Could you check a few things on this drawing? It's one solid part, dimensions in mm from its lowest x, y, z. A direction names the side the tool comes from. Coordinates: 2 decimals unless noted, no trailing zeros. Loops run counter-clockwise (first coordinate to the right, second up) from the corner with the lowest first, then second, coordinate; pieces in that order, holes last. Notation, with made-up numbers: M -38.75,-29 L -26.75,-29 A16 ccw -26.75,-8 Z; hole C -2.75,-16 d11. An arc over 180 degrees is marked long. Use one line per item in the form item = value. Start each with the question number.
(1) Imagine slicing it at A-A, the plane z = 10. Please give me the cut outline in (x, y), and give its area (3 significant figures).
(2) Please list where these lines run through material, in increasing order: L1, parallel to Y at x = 7.07, z = 31.5; L2, parallel to Y at x = 8.75, z = 38; L3, parallel to Y at x = 5.75, z = 27.
(3) Will these pins go through, and if not, where does the flat tip stop? P1, Ø2, axis at x = 12, z = 11.5, coming from the -Y side; P2, Ø1.5, axis at x = 8, z = 21, coming from the -Y side; P3, Ø2, axis at x = 3, z = 10, coming from the -Y side.
(4) Thinking about a two-plate mould opening in X: for the marked faces 3, 4 and 5, which applies, +X half, -X half, draft (parallel to the pull), parting line (faces both ways), or undercut?
(5) Imagine slicing it at C-C, the plane x = 4.5. Please give me the cut outline in (y, z).
(6) On a 3-axis mill with a long thin cutter (end or side, diameter ignored), from which of +Z, -Z, +X, -X, +Y, -Y can I reach the whole of each face in a straight line? I mean the marked faces 1 and 2. Say none if no direction works.
(7) Imagine slicing it at B-B, the plane y = 12.75. Please give me the cut outline in (x, z), and give its area (3 significant figures).
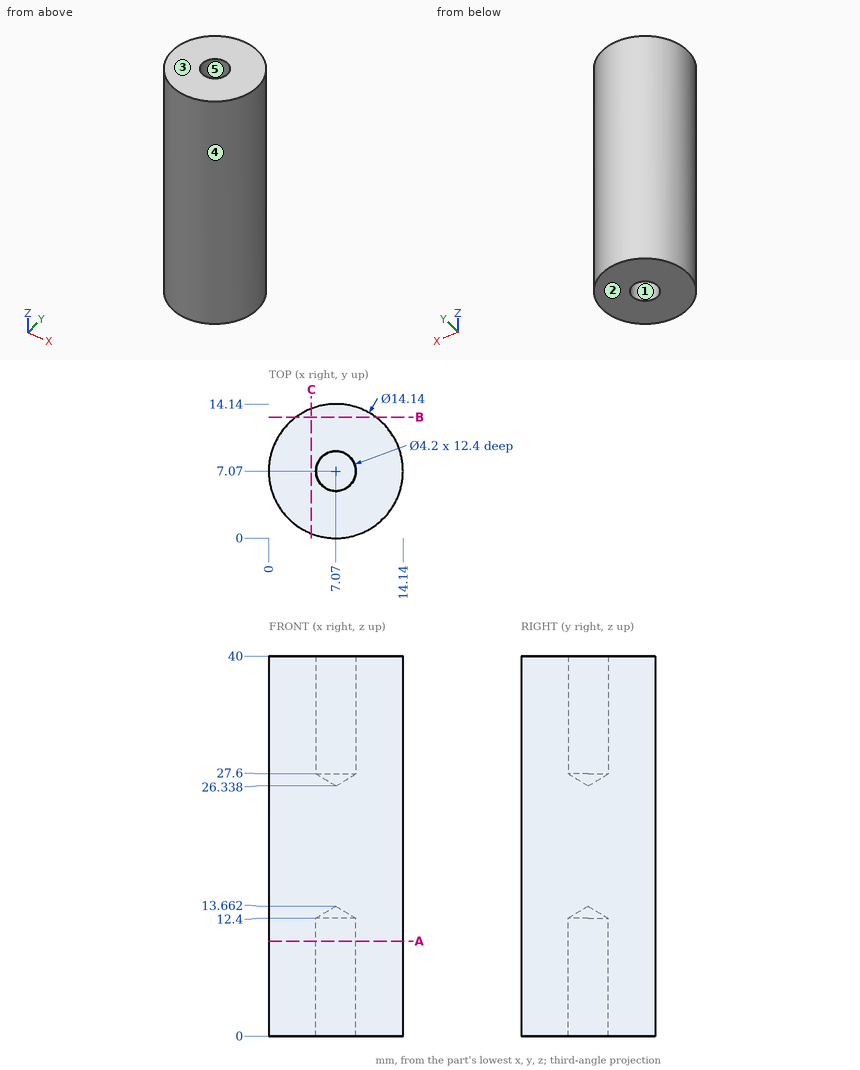
Answer:
q1.outline = C 7.07,7.07 d14.14; hole C 7.07,7.07 d4.2
q1.area = 143 mm²
q2.L1 = 0 to 4.97, 9.17 to 14.14
q2.L2 = 0.2 to 5.81, 8.33 to 13.94
q2.L3 = 0.12 to 14.02
q3.P1 = 1.19
q3.P2 = 0
q3.P3 = 0.7
q4.face_3 = draft
q4.face_4 = parting line
q4.face_5 = undercut
q5.outline = M 0.48,0 L 13.66,0 L 13.66,40 L 0.48,40 Z
q6.face_1 = -Z
q6.face_2 = -Z, +X, -X, +Y, -Y
q7.outline = M 2.86,0 L 11.28,0 L 11.28,40 L 2.86,40 Z
q7.area = 337 mm²
